Can you work these out from the model? Positions are in its coordinate system, mm. Give positions to 0.01 mm unless a question says otherwise; leave off trailing zeros. Loops run counter-clockwise (first coordinate to the right, second up) from the corner with the lowest first, then second, coordinate; pieces in that order, holes last. Notation, with made-up numbers: M 6.25,40 L 59.25,40 A33 cw 59.25,73 Z; hole C 34,82.25 d3. An arc over 180 degrees is marked long. Answer as a JSON object with one key per item and string values.
```python
from build123d import *

# Parameters (mm, degrees)
SKETCH1_W              = 67.564
SKETCH1_H              = 55.88
BOSS_EXTRUDE1_DEPTH    = 17.78
SPLIT1_SURFACE_1_BACK  = 90.463
SPLIT1_SURFACE_1_DEPTH = 180.926


with BuildPart() as part:
    # Sketch1 → Boss-Extrude1 (new body)
    with BuildSketch(Plane.XY):
        Rectangle(SKETCH1_W, SKETCH1_H)
    extrude(amount=BOSS_EXTRUDE1_DEPTH)

    # Split1: cut with a surface, the side it looks to stays
    # Split1 surface: a surface, the sketch's curves swept straight by 180.926 mm
    with BuildLine(Plane(origin=(33.782, 0, 0), x_dir=(0, 0, -1), z_dir=(1, 0, 0)).offset(-SPLIT1_SURFACE_1_BACK), mode=Mode.PRIVATE) as split1_surface_1_path:
        ThreePointArc((-1.685204779, 12.572022866), (-8.89, 26.67), (-16.094795221, 12.572022866))
        ThreePointArc((-16.094795221, 12.572022866), (-15.296445708, 8.89), (-16.094795221, 5.207977134))
        ThreePointArc((-16.094795221, 5.207977134), (-17.78, 0), (-16.094795221, -5.207977134))
        ThreePointArc((-16.094795221, -5.207977134), (-15.296445708, -8.89), (-16.094795221, -12.572022866))
        ThreePointArc((-16.094795221, -12.572022866), (-8.89, -26.67), (-1.685204779, -12.572022866))
        ThreePointArc((-1.685204779, -12.572022866), (-2.483554292, -8.89), (-1.685204779, -5.207977134))
        ThreePointArc((-1.685204779, -5.207977134), (0, 0), (-1.685204779, 5.207977134))
        ThreePointArc((-1.685204779, 5.207977134), (-2.483554292, 8.89), (-1.685204779, 12.572022866))
    split1_surface_1 = Shell.extrude(split1_surface_1_path.wire(), (1 * SPLIT1_SURFACE_1_DEPTH, 0 * SPLIT1_SURFACE_1_DEPTH, 0 * SPLIT1_SURFACE_1_DEPTH))
    split(bisect_by=split1_surface_1, keep=Keep.TOP)


solid = part.part
```
1) Suppose I cut it at C-C, the plane z = 13.5. Write out the boundary of the cut face in (x, y).
Answer list:
{"outline": "M -33.78,-25.38 L 33.78,-25.38 L 33.78,25.38 L -33.78,25.38 Z"}
2) Suppose I cut it at A-A, the plane x = -30. Write out the boundary of the cut face in (y, z), and give its area (3 significant figures).
Answer list:
{"outline": "M -12.57,1.69 A8.89 cw -5.21,1.69 A8.89 ccw 5.21,1.69 A8.89 cw 12.57,1.69 A8.89 ccw long 12.57,16.09 A8.89 cw 5.21,16.09 A8.89 ccw -5.21,16.09 A8.89 cw -12.57,16.09 A8.89 ccw long Z", "area": "793 mm^2"}
3) If we mould it in two halves opening along Y, with no side actions, what happens to faces 1 (the flat face through (33.782, 0, 9)), 2 (the cylindrical face through (-0.473, -8.837, 15.297))? For each: +Y half, -Y half, draft (parallel to the pull), parting line (faces both ways), or undercut.
Answer list:
{"face 1": "draft", "face 2": "undercut"}
4) Suppose I cut it at B-B, the plane y = -23. Write out the boundary of the cut face in (x, z), and give its area (3 significant figures).
Answer list:
{"outline": "M -33.78,1.69 L 33.78,1.69 L 33.78,16.09 L -33.78,16.09 Z", "area": "972 mm^2"}
5) Please list where these lines run through material, in increasing order: line 1 along Z through (x, y) = (23.5, 23); line 2 along Z through (x, y) = (1, 9); line 3 along Y through (x, z) = (24, 8.5). Write a range as from..to.
Answer list:
{"line 1": "1.69..16.09", "line 2": "2.48..15.3", "line 3": "-26.66..26.66"}
